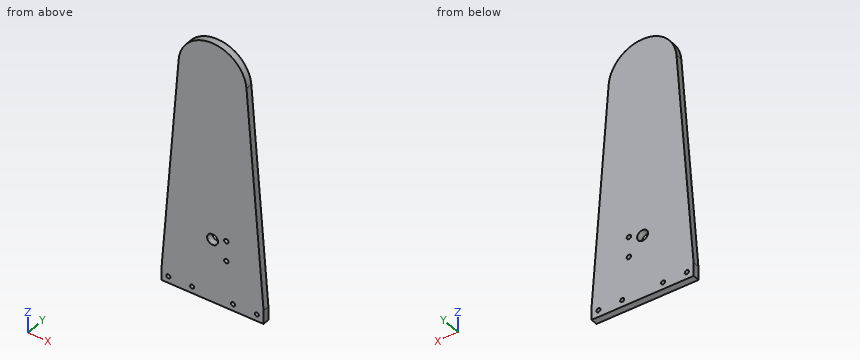
from build123d import *

# Parameters (mm, degrees)
SKETCH_1_R      = 1.5
SKETCH_1_R_2    = 4
SKETCH_1_R_3    = 1.6
EXTRUDE_1_DEPTH = 5


with BuildPart() as part:
    # ｽｹｯﾁ1 → ﾎﾞｽ - 押し出し1 (new body)
    with BuildSketch(Plane(origin=(0, 0, 0), x_dir=(1, 0, 0), z_dir=(0, 1, 0))):
        with BuildLine():
            Line((0, 0), (0, -10))
            Line((0, -10), (12.575038747, -171.935537794))
            ThreePointArc((12.575038747, -171.935537794), (37.5, -195), (62.424961253, -171.935537794))
            Line((62.424961253, -171.935537794), (75, -10))
            Line((75, -10), (75, 0))
            Line((75, 0), (0, 0))
        make_face()
        with Locations(Location((5, -5, 0), (0, 0, 270))):
            Circle(SKETCH_1_R, mode=Mode.SUBTRACT)
        with Locations(Location((70, -5, 0), (0, 0, 90))):
            Circle(SKETCH_1_R, mode=Mode.SUBTRACT)
        with Locations(Location((22.5, -5, 0), (0, 0, 270))):
            Circle(SKETCH_1_R, mode=Mode.SUBTRACT)
        with Locations(Location((52.5, -5, 0), (0, 0, 90))):
            Circle(SKETCH_1_R, mode=Mode.SUBTRACT)
        with Locations(Location((37.5, -47.1, 0), (0, 0, 270))):
            Circle(SKETCH_1_R_2, mode=Mode.SUBTRACT)
        with Locations(Location((47.6, -35.3, 0), (0, 0, 270))):
            Circle(SKETCH_1_R_3, mode=Mode.SUBTRACT)
        with Locations(Location((47.6, -50.3, 0), (0, 0, 270))):
            Circle(SKETCH_1_R_3, mode=Mode.SUBTRACT)
    extrude(amount=EXTRUDE_1_DEPTH)


solid = part.part
The model under review builds one solid part; all positions refer to its coordinate system, in mm. Round coordinates to 2 decimals unless told otherwise and drop trailing zeros. Loops run counter-clockwise (first coordinate to the right, second up) from the corner with the lowest first, then second, coordinate; pieces in that order, holes last. Notation, with made-up numbers: (-33, -28.5) -> (26, -28.5) arc R30 cw to (26, 4.5) -> close; hole circle Ø1 at (31, 9.25). An arc over 180 degrees is marked (long way). Write item = value, one per line. Start each with the question number.
Item 1: To check wall thickness, follow L1, parallel to X at y = 3.1, z = 5; L2, parallel to X at y = 2.2, z = 50.3; L3, parallel to Z at x = 46.5, y = 4.3. State the ranges of each line that lie inside material, in increasing order.
Item 2: Take a section at A-A on x = 37.5. Give the boundary of the cut face in (y, z).
Item 3: Take a section at C-C on z = 45. Give the boundary of the cut face in (x, y), plus the area to 3 significant figures.
Item 4: Insertion check: pin 1 (2.5 mm diameter, centred on x = 52.5, z = 5, fed in from +Y); pin 2 (2 mm diameter, centred on x = 17, y = 3.5, fed in from +Z); pin 3 (2 mm diameter, centred on y = 2, z = 129, fed in from -X). Each pin has a flat end and moves straight along its axis. Give the tip position at first contact, or say it passes through.
Item 5: Take a section at D-D on z = 159.5. Give the boundary of the cut face in (x, y), plus the area to 3 significant figures.
Item 6: Take a section at B-B on y = 1.3. Give the boundary of the cut face in (x, z), plus the area to 3 significant figures.
Result:
q1.L1 = 0 to 3.5, 6.5 to 21, 24 to 51, 54 to 68.5, 71.5 to 75
q1.L2 = 3.13 to 35.1, 39.9 to 46, 49.2 to 71.87
q1.L3 = 0 to 34.14, 36.46 to 49.14, 51.46 to 193.32
q2.outline = (0, 0) -> (5, 0) -> (5, 43.1) -> (0, 43.1) -> close; (0, 51.1) -> (5, 51.1) -> (5, 195) -> (0, 195) -> close
q3.outline = (2.72, 0) -> (34.1, 0) -> (34.1, 5) -> (2.72, 5) -> close; (40.9, 0) -> (72.28, 0) -> (72.28, 5) -> (40.9, 5) -> close
q3.area = 314 mm²
q4.pin_1 = through
q4.pin_2 = 185.64
q4.pin_3 = 9.16
q5.outline = (11.61, 0) -> (63.39, 0) -> (63.39, 5) -> (11.61, 5) -> close
q5.area = 259 mm²
q6.outline = (0, 0) -> (75, 0) -> (75, 10) -> (62.42, 171.94) arc R25 ccw to (12.58, 171.94) -> (0, 10) -> close; hole circle Ø3 at (5, 5); hole circle Ø3 at (22.5, 5); hole circle Ø8 at (37.5, 47.1); hole circle Ø3.2 at (47.6, 35.3); hole circle Ø3.2 at (47.6, 50.3); hole circle Ø3 at (52.5, 5); hole circle Ø3 at (70, 5)
q6.area = 11,600 mm²
